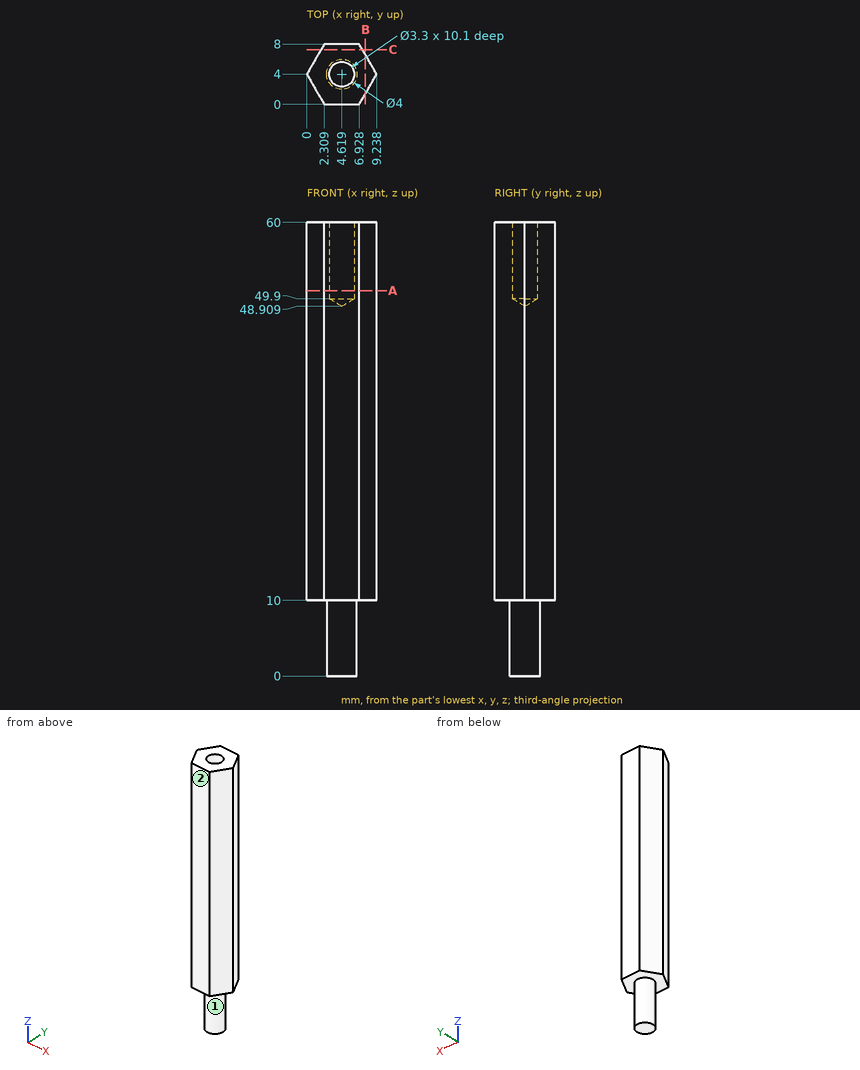
Answer from the drawing. Dimensions are ordinates in mm from the lowest x, y and z of the part. A direction names the side the tool comes from. Give positions to 0.01 mm unless a question says otherwise; leave off trailing zeros. Write each loop counter-clockwise with the first axis right and the second up, starting at its lowest first coordinate (ties: lowest second). Pieces come first, ordered by that corner, then holes.
1) Given P1, Ø2.5, axis at x = 4.62, y = 4, coming from the -Z side; P2, Ø3, axis at y = 6, z = 11, coming from the +X side, each flat-ended and moving along its own axis, determine where each tip first touches the part or whether it passes through.
2) Section A-A (z = 51) is taken. Write down the section's boundary in (x, y).
3) Section C-C (y = 7.25) is taken. Write down the section's boundary in (x, z), and give its area (3 significant figures).
4) Find the intervals of material crossed by L1, parallel to X at y = 4, z = 54.75; L2, parallel to Z at x = 6.5, y = 6.5; L3, parallel to Y at x = 6, z = 57.5 (1 decimal), in increasing order.
5) Section B-B (x = 7.75) is taken. Write down the section's boundary in (y, z), and give its area (3 significant figures).
6) A tool of negligible diameter and unlimited length cuts with its end or side. For the marked faces 1 and 2, from which of +Z, -Z, +X, -X, +Y, -Y can it reach the whole face along a straight path? Write none if from no direction.
Response:
1. P1: stops at z = 0
1. P2: stops at x = 8.95
2. outline: (0, 4) - (2.31, 0) - (6.93, 0) - (9.24, 4) - (6.93, 8) - (2.31, 8) - close; hole circle Ø3.3 at (4.62, 4)
3. outline: (1.88, 10) - (7.36, 10) - (7.36, 60) - (1.88, 60) - close
3. area: 274 mm2
4. L1: x = 0 to 2.97, 6.27 to 9.24
4. L2: z = 10 to 60
4. L3: y = 0 to 3.1, 4.9 to 8
5. outline: (1.42, 10) - (6.58, 10) - (6.58, 60) - (1.42, 60) - close
5. area: 258 mm2
6. face 1: -Z
6. face 2: +Z, -Z, +X, -X, -Y
